The listing builds one solid part. Answer for the finished solid, in the listing's coordinates (mm). A direction names the side the tool comes from. Round coordinates to 2 decimals unless told otherwise and drop trailing zeros. Write each loop counter-clockwise with the first axis right and the second up, starting at its lowest first coordinate (ties: lowest second). Pieces come first, ordered by that corner, then holes. Notation, with made-up numbers: M 5.5,20 L 47.5,20 A25 ccw 47.5,47 Z; hole C 3,88.5 d5. An arc over 180 degrees is marked long. Write each question's results on one line, items separated by ' | '.
from build123d import *

# Parameters (mm, degrees)
BOSS_EXTRUDE1_DEPTH        = 10
BOSS_EXTRUDE1_DEPTH_BACK   = 10
SKETCH4_R                  = 20
SKETCH4_R_2                = 10
BOSS_EXTRUDE1_2_DEPTH      = 10
BOSS_EXTRUDE1_2_DEPTH_BACK = 10
SKETCH6_R                  = 7
BOSS_EXTRUDE2_DEPTH        = 20
FILLET1_R                  = 3


with BuildPart() as part:
    # Sketch4 → Boss-Extrude1 (new, two sides: drawn at the far end of the back side and taken through both)
    with BuildSketch(Plane(origin=(0, 0, 0), x_dir=(1, 0, 0), z_dir=(0, 1, 0)).offset(-BOSS_EXTRUDE1_DEPTH_BACK)):
        with Locations(Location((0, 0, 0), (0, 0, 270))):
            Circle(SKETCH4_R)
        with Locations(Location((0, 0, 0), (0, 0, 270))):
            Circle(SKETCH4_R_2, mode=Mode.SUBTRACT)
    extrude(amount=BOSS_EXTRUDE1_DEPTH + BOSS_EXTRUDE1_DEPTH_BACK)



with BuildPart() as body_2:
    # Sketch4 → Boss-Extrude1 2 (new, two sides: drawn at the far end of the back side and taken through both)
    with BuildSketch(Plane(origin=(0, 0, 0), x_dir=(1, 0, 0), z_dir=(0, 1, 0)).offset(-BOSS_EXTRUDE1_2_DEPTH_BACK)):
        with BuildLine():
            Line((-10, -35), (10, -35))
            Line((10, -35), (10, -70))
            ThreePointArc((10, -70), (30, -90), (50, -70))
            ThreePointArc((50, -70), (55, -65), (60, -70))
            ThreePointArc((60, -70), (49.38848107, -104.36409372), (17, -120))
            Line((17, -120), (-17, -120))
            ThreePointArc((-17, -120), (-49.38848107, -104.36409372), (-60, -70))
            ThreePointArc((-60, -70), (-55, -65), (-50, -70))
            ThreePointArc((-50, -70), (-30, -90), (-10, -70))
            Line((-10, -70), (-10, -35))
        make_face()
    extrude(amount=BOSS_EXTRUDE1_2_DEPTH + BOSS_EXTRUDE1_2_DEPTH_BACK)


with BuildPart() as part_1:
    add(part.part)

    add(body_2.part)  # Boss-Extrude2 merges body 2
    # Sketch6 → Boss-Extrude2 (add)
    with BuildSketch(Plane(origin=(0, 0, 35), x_dir=(-1, 0, 0), z_dir=(0, 0, -1))):
        with Locations(Location((0, 0, 0), (0, 0, 180))):
            Circle(SKETCH6_R)
    extrude(amount=BOSS_EXTRUDE2_DEPTH)

    # Fillet1
    fillet1_edges = [part_1.edges().sort_by_distance(p)[0] for p in [
        (-7, 0, 35),
    ]]
    fillet(fillet1_edges, radius=FILLET1_R - 0.0001)  # a hair under: the kernel refuses the full size


solid = part_1.part
1) The mould has two halves that part along Z. Classify faces 1 (the face through (-55, 0, 65)), 2 (the face through (9, 10, -5)), 3 (the face through (-6, -8.2, 35)): +Z half, -Z half, draft (parallel to the pull), parting line (faces both ways), or undercut.
Return value:
face 1: -Z half | face 2: draft | face 3: undercut
2) Section B-B (z = 0) is taken. Determine the outline of the cut face in (x, y).
Return value:
outline: M -20,-10 L -10,-10 L -10,10 L -20,10 Z; M 10,-10 L 20,-10 L 20,10 L 10,10 Z
3) A tool of negligible diameter and unlimited length cuts with its end or side. For faces 4 (the face through (30, 0, 90)), 5 (the face through (-7, 0, 25)), 6 (the face through (1, -10, 86)), from which of +Z, -Z, +X, -X, +Y, -Y can it reach the whole face along a straight path? Write none if from no direction.
Return value:
face 4: +Y, -Y | face 5: none | face 6: +Z, -Z, +X, -X, -Y
4) Section C-C (z = 76) is taken. Determine the outline of the cut face in (x, y), then the cut area to 3 significant figures.
Return value:
outline: M -60.27,-10 L -49.08,-10 L -49.08,10 L -60.27,10 Z; M -10.92,-10 L 10.92,-10 L 10.92,10 L -10.92,10 Z; M 49.08,-10 L 60.27,-10 L 60.27,10 L 49.08,10 Z | area: 884 mm²
5) Find the intervals of material crossed by line 1 (X direction, y = -0.75, z = 0); line 2 (X direction, y = 6.5, z = 75); line 3 (X direction, y = -1.5, z = 86.5), in increasing order.
Return value:
line 1: -20 to -10, 10 to 20 | line 2: -60.28 to -49.36, -10.64 to 10.64, 49.36 to 60.28 | line 3: -58.79 to -41.3, -18.7 to 18.7, 41.3 to 58.79
6) Each of these flat-tipped pins is pushed along its axis until it touches: pin 1 (5 mm diameter, centred on x = 8, y = 8, fed in from -Z); pin 2 (1.5 mm diameter, centred on y = -6.5, z = 101, fed in from -X); pin 3 (6 mm diameter, centred on y = 1.5, z = 52, fed in from +X); pin 4 (4 mm diameter, centred on y = 1, z = 76, fed in from +X). Where does it stop, or does it pass through?
Return value:
pin 1: z = -19.23 | pin 2: x = -52.53 | pin 3: x = 10 | pin 4: x = 60.28
7) Section D-D (y = 8.5) is taken. State how many separate pieces and enclosed holes the cut face has, then the cut area to 3 significant figures.
Return value:
separate pieces: 2 | enclosed holes: 1 | area: 5,630 mm²
